from build123d import *

# Parameters (mm, degrees)
SKETCH1_W           = 160
SKETCH1_H           = 160
BOSS_EXTRUDE1_DEPTH = 2
SKETCH2_R           = 5
CUT_EXTRUDE1_DEPTH  = 2
SKETCH5_R           = 1.6
CUT_EXTRUDE3_DEPTH  = 2
SKETCH8_R           = 3
SKETCH8_R_2         = 1.6
CUT_EXTRUDE5_DEPTH  = 2


with BuildPart() as part:
    # Sketch1 → Boss-Extrude1 (new body)
    with BuildSketch(Plane.XY):
        Rectangle(SKETCH1_W, SKETCH1_H)
    extrude(amount=BOSS_EXTRUDE1_DEPTH)

    # Sketch2 → Cut-Extrude1 (cut)
    with BuildSketch(Plane.XY.offset(2)):
        Circle(SKETCH2_R)
    extrude(amount=-CUT_EXTRUDE1_DEPTH, mode=Mode.SUBTRACT)

    # Sketch5 → Cut-Extrude3 (cut)
    with BuildSketch(Plane(origin=(0, 0, 0), x_dir=(-1, 0, 0), z_dir=(0, 0, -1))):
        with Locations((10.5, 10.5)):
            Circle(SKETCH5_R)
        with Locations((10.5, -10.5)):
            Circle(SKETCH5_R)
        with Locations((-10.5, -10.5)):
            Circle(SKETCH5_R)
        with Locations((-10.5, 10.5)):
            Circle(SKETCH5_R)
    extrude(amount=-CUT_EXTRUDE3_DEPTH, mode=Mode.SUBTRACT)

    # Sketch8 → Cut-Extrude5 (cut)
    with BuildSketch(Plane(origin=(0, 0, 0), x_dir=(-1, 0, 0), z_dir=(0, 0, -1))):
        with Locations((54, 0)):
            Circle(SKETCH8_R)
        with Locations((54, 12.5)):
            Circle(SKETCH8_R_2)
        with Locations((64.825317547, 6.25)):
            Circle(SKETCH8_R_2)
        with Locations((64.825317547, -6.25)):
            Circle(SKETCH8_R_2)
        with Locations((54, -12.5)):
            Circle(SKETCH8_R_2)
        with Locations((43.174682453, -6.25)):
            Circle(SKETCH8_R_2)
        with Locations((43.174682453, 6.25)):
            Circle(SKETCH8_R_2)
    extrude(amount=-CUT_EXTRUDE5_DEPTH, mode=Mode.SUBTRACT)


solid = part.part
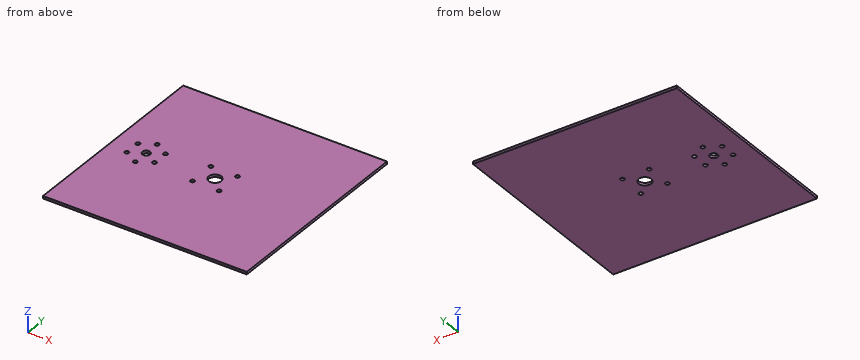
The model under review builds one solid part; all positions refer to its coordinate system, in mm. Coordinates: 2 decimals unless noted, no trailing zeros. Write each loop counter-clockwise with the first axis right and the second up, starting at its lowest first coordinate (ties: lowest second). Pieces come first, ordered by that corner, then holes. Notation, with made-up numbers: (-5, -18) - (5, -18) arc R20 cw to (5, 2) - close; hole circle Ø2 at (-35.5, 39). An arc over 180 degrees is marked (long way). Answer as CSV lines item,"result".
(1) We need section B-B (x = 0). Give the boundary of the cut face in (y, z).
Data:
outline,"(-80, 0) - (-5, 0) - (-5, 2) - (-80, 2) - close; (5, 0) - (80, 0) - (80, 2) - (5, 2) - close"
(2) For line 1 along Y through (x, z) = (11.5, 0.4); line 2 along X through (y, z) = (-1, 0.25); line 3 along X through (y, z) = (10, 0.2), list the stretches that pass through material, from the lowest coordinate up. Write a range as [from, to].
Data:
line 1,"y = [-80, -11.75], [-9.25, 9.25], [11.75, 80]"
line 2,"x = [-80, -56.83], [-51.17, -4.9], [4.9, 80]"
line 3,"x = [-80, -12.02], [-8.98, 8.98], [12.02, 80]"
(3) We need section A-A (y = 0). Give the boundary of the cut face in (x, z).
Data:
outline,"(-80, 0) - (-57, 0) - (-57, 2) - (-80, 2) - close; (-51, 0) - (-5, 0) - (-5, 2) - (-51, 2) - close; (5, 0) - (80, 0) - (80, 2) - (5, 2) - close"
